Part model, mm, in its own coordinate system. A direction names the side the tool comes from. Coordinates: 2 decimals unless noted, no trailing zeros. Order: outer loops, then holes, each group sorted by start corner. A loop starts at its lowest first (then second) coordinate and runs counter-clockwise, first axis right, second up.
from build123d import *

# Parameters (mm, degrees)
SKETCH_1_R          = 1.75
SKETCH_1_W          = 20.2
SKETCH_1_H          = 40.5
EXTRUDE_1_DEPTH     = 5
SKETCH_2_W          = 10
SKETCH_2_H          = 20
SKETCH_2_H_2        = 70
EXTRUDE_2_DEPTH     = 15
SKETCH_3_R          = 4
CUT_EXTRUDE_1_DEPTH = 146
FILLET_1_R          = 10


with BuildPart() as part:
    # 草图1 → 凸台-拉伸1 (new body)
    with BuildSketch(Plane.XY):
        with BuildLine():
            Line((35, -75), (-35, -75))
            ThreePointArc((-35, -75), (-38.535533906, -73.535533906), (-40, -70))
            Line((-40, -70), (-40, 70))
            ThreePointArc((-40, 70), (-38.535533906, 73.535533906), (-35, 75))
            Line((-35, 75), (35, 75))
            ThreePointArc((35, 75), (38.535533906, 73.535533906), (40, 70))
            Line((40, 70), (40, -70))
            ThreePointArc((40, -70), (38.535533906, -73.535533906), (35, -75))
        make_face()
        with Locations((-5, -22)):
            Circle(SKETCH_1_R, mode=Mode.SUBTRACT)
        with Locations(Location((5, -22, 0), (0, 0, 180))):
            Circle(SKETCH_1_R, mode=Mode.SUBTRACT)
        with Locations((5, -70)):
            Circle(SKETCH_1_R, mode=Mode.SUBTRACT)
        with Locations(Location((-5, -70, 0), (0, 0, 180))):
            Circle(SKETCH_1_R, mode=Mode.SUBTRACT)
        with Locations((0, -46)):
            Rectangle(SKETCH_1_W, SKETCH_1_H, mode=Mode.SUBTRACT)
    extrude(amount=EXTRUDE_1_DEPTH)

    # 草图2 → 凸台-拉伸2 (add)
    with BuildSketch(Plane.XY.offset(5)):
        with Locations((20, 55)):
            Rectangle(SKETCH_2_W, SKETCH_2_H)
        with Locations((30, -25)):
            Rectangle(SKETCH_2_W, SKETCH_2_H_2)
        with Locations((-30, -25)):
            Rectangle(SKETCH_2_W, SKETCH_2_H_2)
        with Locations((-20, 55)):
            Rectangle(SKETCH_2_W, SKETCH_2_H)
    extrude(amount=EXTRUDE_2_DEPTH)

    # 草图3 → 切除-拉伸1 (cut)
    with BuildSketch(Plane.ZY.offset(35)):
        with Locations((12.5, 55)):
            Circle(SKETCH_3_R)
        with BuildLine():
            Line((8.5, -50), (8.5, 0))
            ThreePointArc((8.5, 0), (12.5, 4), (16.5, 0))
            Line((16.5, 0), (16.5, -50))
            ThreePointArc((16.5, -50), (12.5, -54), (8.5, -50))
        make_face()
    extrude(amount=-CUT_EXTRUDE_1_DEPTH, mode=Mode.SUBTRACT)

    # 圆角1
    fillet_1_edges = [part.edges().sort_by_distance(p)[0] for p in [
        (30, -60, 20),
        (-30, -60, 20),
        (30, 10, 20),
        (-30, 10, 20),
        (20, 45, 20),
        (20, 65, 20),
        (-20, 45, 20),
        (-20, 65, 20),
    ]]
    fillet(fillet_1_edges, radius=FILLET_1_R - 0.0001)  # a hair under: the kernel refuses the full size


solid = part.part
Q1. Mould opens along Z. For faces 1 (the face through (-30.1, -54, 12.6)), 2 (the face through (-30.1, 4, 12.4)), 3 (the face through (40, 1, 2)), 4 (the face through (-19.93, 47.85, 16.99)) say: pulls with the +Z half, pulls with the -Z half, needs draft (parallel to the pull), parting line crosses it, or undercut.
Results list:
face 1: undercut
face 2: undercut
face 3: needs draft
face 4: pulls with the +Z half
Q2. Cut at A-A on x = 5. Write the cut outline in (y, z).
Results list:
outline: (-75, 0) - (-71.75, 0) - (-71.75, 5) - (-75, 5) - close; (-68.25, 0) - (-66.25, 0) - (-66.25, 5) - (-68.25, 5) - close; (-25.75, 0) - (-23.75, 0) - (-23.75, 5) - (-25.75, 5) - close; (-20.25, 0) - (75, 0) - (75, 5) - (-20.25, 5) - close
Q3. Wall check: line 1 along Y through (x, z) = (-5, 3.6); line 2 along X through (y, z) = (-70, 1.3); line 3 along X through (y, z) = (-55, 15.75). Give the ranges that are in metal, low to high.
Results list:
line 1: y = -75 to -71.75, -68.25 to -66.25, -25.75 to -23.75, -20.25 to 75
line 2: x = -40 to -6.75, -3.25 to 3.25, 6.75 to 40
line 3: x = -35 to -25, 25 to 35
Q4. Pin check, flat tips, straight feed: pin 1 Ø7.5 at (y, z) = (-28.5, 10.5) entering from -X; pin 2 Ø1.5 at (y, z) = (2, 8.5) entering from +X; pin 3 Ø4 at (x, y) = (-5, -70) entering from -Z; pin 4 Ø10.5 at (y, z) = (55, 12.5) entering from -X. Stop position of each tip, or through.
Results list:
pin 1: stops at x = -35
pin 2: stops at x = 35
pin 3: stops at z = 0
pin 4: stops at x = -25
Q5. Cut at D-D on z = 12.5. Count the separate pieces of the cut face and the enclosed holes in it, and give its area (3 significant figures).
Results list:
separate pieces: 8
enclosed holes: 0
area: 455 mm2
Q6. Which spindle directions (+Z, -Z, +X, -X, +Y, -Y) get a long thin tool onto all of the face, cutting with end or side? Do faces 5 (the face through (-30, -25, 20)), 6 (the face through (35, -25, 7)), 7 (the face through (29.9, 4, 12.4)), 8 (the face through (0, -25.75, 2)), 9 (the face through (-20, 65, 7)). Say none if no direction does.
Results list:
face 5: +Z, +X, -X, +Y, -Y
face 6: +Z, +X, +Y, -Y
face 7: +X, -X
face 8: +Z, -Z
face 9: +Z, +X, -X, +Y
Q7. Cut at C-C on y = -22. Write the cut outline in (x, z), and give its area (3 significant figures).
Results list:
outline: (-40, 0) - (-6.75, 0) - (-6.75, 5) - (-25, 5) - (-25, 8.5) - (-35, 8.5) - (-35, 5) - (-40, 5) - close; (-35, 16.5) - (-25, 16.5) - (-25, 20) - (-35, 20) - close; (-3.25, 0) - (3.25, 0) - (3.25, 5) - (-3.25, 5) - close; (6.75, 0) - (40, 0) - (40, 5) - (35, 5) - (35, 8.5) - (25, 8.5) - (25, 5) - (6.75, 5) - close; (25, 16.5) - (35, 16.5) - (35, 20) - (25, 20) - close
area: 505 mm2
